Design review of the part built by this model. Coordinates are the model's own, in mm. Coordinates: 2 decimals unless noted, no trailing zeros. Loops run counter-clockwise (first coordinate to the right, second up) from the corner with the lowest first, then second, coordinate; pieces in that order, holes last. Notation, with made-up numbers: (-27, 58) - (-4, 58) arc R22 ccw to (-4, 69) - close; hole circle Ø3 at (20, 77). An arc over 180 degrees is marked (long way). Answer in a Markdown table with one row per item. Add a question column.
(1) We need section A-A, the plane x = 33. Write out the cut boundary in (y, z), plus the area to 3 significant figures.
(2) We need section C-C, the plane y = 0. Write out the cut boundary in (x, z), plus the area to 3 significant figures.
(3) To check wall thickness, follow L1, parallel to Y at x = 28, z = 1.9; L2, parallel to X at y = -6, z = 1.5; L3, parallel to X at y = -2, z = 0.95. State the ranges of each line that lie inside material, in increasing order. Write a range as [from, to].
(4) Clearance check with flat-ended pins moving along their axes: pin 1 (20 mm diameter, centred on x = 28.21, y = -6.41, fed in from +Z); pin 2 (1.1 mm diameter, centred on y = 11, z = 0.5, fed in from +X). State where each tip first meets the part, or that it passes through.
(5) We need section B-B, the plane z = 0.4. Write out the cut boundary in (x, y), plus the area to 3 significant figures.
(6) The part is to be moulded in two halves that separate along X. For faces 1 (the face through (82, -6, 0)), 2 (the face through (155.357, -18.399, 1.07)), 3 (the face through (144.24, -9.45, 1.07)), say which applies: released by +X, released by -X, zero draft, split by the parting line, or undercut.
(7) We need section D-D, the plane x = 108. Write out the cut boundary in (y, z).
from build123d import *

# Parameters (mm, degrees)
CROQUIS1_R              = 1.55
SALIENTE_EXTRUIR1_DEPTH = 2.11
CROQUIS5_R              = 11
CORTAR_EXTRUIR1_DEPTH   = 2.11
CROQUIS6_R              = 5
CORTAR_EXTRUIR2_DEPTH   = 2.11
REDONDEO1_R             = 10


with BuildPart() as part:
    # Croquis1 → Saliente-Extruir1 (new body)
    with BuildSketch(Plane.XY):
        Polygon((158.208826457, -21.405767977), (158.208826457, 8.594232023), (48.708826457, 8.594232023), (48.708826457, 14.094232023), (7.708826457, 14.094232023), (7.708826457, -26.905767977), (48.708826457, -26.905767977), (48.708826457, -21.405767977), align=None)
        with Locations((12.708826457, -21.905767977)):
            Circle(CROQUIS1_R, mode=Mode.SUBTRACT)
        with Locations((12.708826457, 9.094232023)):
            Circle(CROQUIS1_R, mode=Mode.SUBTRACT)
        with Locations((43.708826457, 9.094232023)):
            Circle(CROQUIS1_R, mode=Mode.SUBTRACT)
        with Locations((43.708826457, -21.905767977)):
            Circle(CROQUIS1_R, mode=Mode.SUBTRACT)
    extrude(amount=SALIENTE_EXTRUIR1_DEPTH)

    # Croquis5 → Cortar-Extruir1 (cut)
    with BuildSketch(Plane.XY.offset(2.11)):
        with Locations((28.208826457, -6.405767977)):
            Circle(CROQUIS5_R)
    extrude(amount=-CORTAR_EXTRUIR1_DEPTH, mode=Mode.SUBTRACT)

    # Croquis6 → Cortar-Extruir2 (cut)
    with BuildSketch(Plane.XY.offset(2.11)):
        with Locations((148.208826457, -6.405767977)):
            Circle(CROQUIS6_R)
    extrude(amount=-CORTAR_EXTRUIR2_DEPTH, mode=Mode.SUBTRACT)

    # Redondeo1
    redondeo1_edges = [part.edges().sort_by_distance(p)[0] for p in [
        (158.208826457, -21.405767977, 1.055),
    ]]
    fillet(redondeo1_edges, radius=REDONDEO1_R)


solid = part.part
Responses:
| question | item | result |
|---|---|---|
| 1 | outline | (-26.91, 0) - (-16.31, 0) - (-16.31, 2.11) - (-26.91, 2.11) - close; (3.5, 0) - (14.09, 0) - (14.09, 2.11) - (3.5, 2.11) - close |
| 1 | area | 44.7 mm2 |
| 2 | outline | (7.71, 0) - (19.27, 0) - (19.27, 2.11) - (7.71, 2.11) - close; (37.15, 0) - (158.21, 0) - (158.21, 2.11) - (37.15, 2.11) - close |
| 2 | area | 280 mm2 |
| 3 | L1 | y = [-26.91, -17.4], [4.59, 14.09] |
| 3 | L2 | x = [7.71, 17.22], [39.2, 143.23], [153.19, 158.21] |
| 3 | L3 | x = [7.71, 18.13], [38.29, 145.84], [150.57, 158.21] |
| 4 | pin 1 | passes through |
| 4 | pin 2 | stops at x = 48.71 |
| 5 | outline | (7.71, -26.91) - (48.71, -26.91) - (48.71, -21.41) - (148.21, -21.41) arc R10 ccw to (158.21, -11.41) - (158.21, 8.59) - (48.71, 8.59) - (48.71, 14.09) - (7.71, 14.09) - close; hole circle Ø3.1 at (12.71, -21.91); hole circle Ø3.1 at (12.71, 9.09); hole circle Ø22 at (28.21, -6.41); hole circle Ø3.1 at (43.71, -21.91); hole circle Ø3.1 at (43.71, 9.09); hole circle Ø10 at (148.21, -6.41) |
| 5 | area | 4,460 mm2 |
| 6 | face 1 | zero draft |
| 6 | face 2 | released by +X |
| 6 | face 3 | undercut |
| 7 | outline | (-21.41, 0) - (8.59, 0) - (8.59, 2.11) - (-21.41, 2.11) - close |
